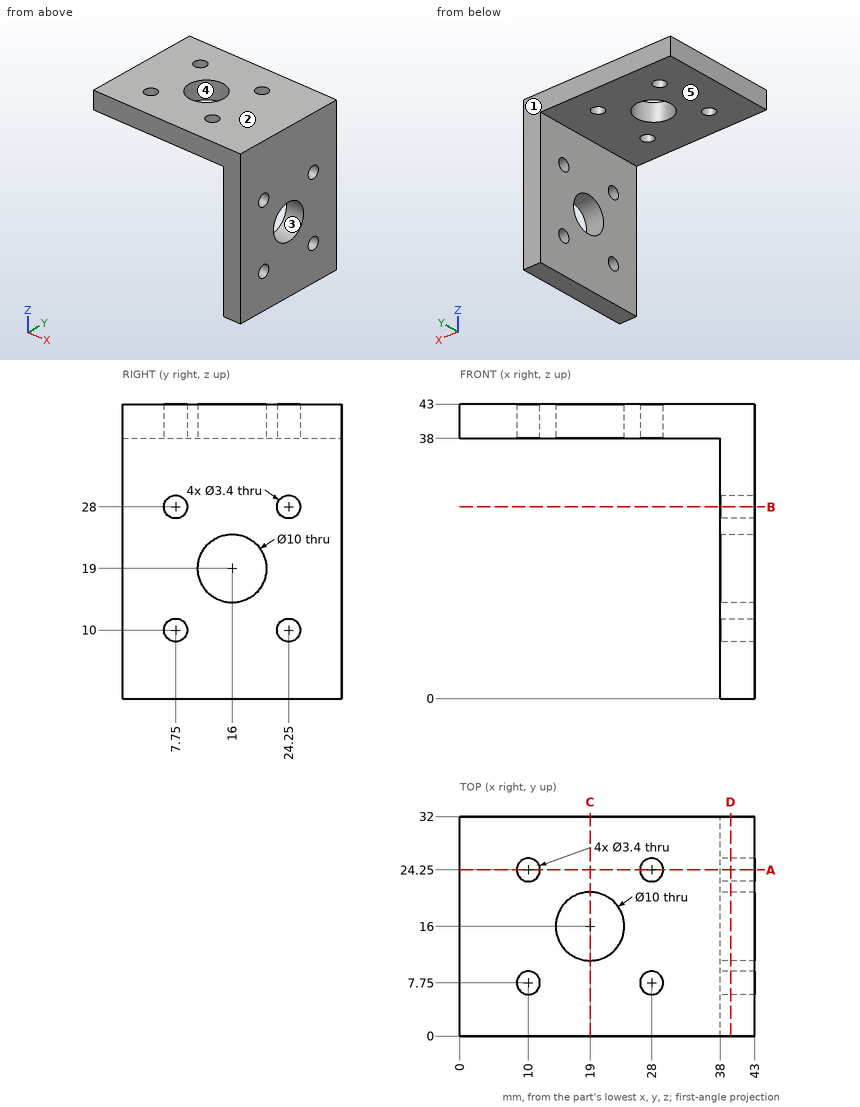
Design review of the part shown in the three views and the two pictorial views. Dimensions are in mm from the part's minimum x, y and z. A direction names the side the tool comes from. Coordinates: 2 decimals unless noted, no trailing zeros. Write each loop counter-clockwise with the first axis right and the second up, starting at its lowest first coordinate (ties: lowest second). Pieces come first, ordered by that corner, then holes. Notation, with made-up numbers: (28, 69.25) -> (51, 69.25) arc R26 ccw to (51, 101.25) -> close; hole circle Ø10 at (43, -23.5). An arc over 180 degrees is marked (long way). Answer in a Markdown table with one row per item.
1. We need section B-B, the plane z = 28. State the section outline as (x, y) points, and give its area (3 significant figures).
Answers below:
| item | result |
|---|---|
| outline | (38, 0) -> (43, 0) -> (43, 6.05) -> (38, 6.05) -> close; (38, 9.45) -> (43, 9.45) -> (43, 22.55) -> (38, 22.55) -> close; (38, 25.95) -> (43, 25.95) -> (43, 32) -> (38, 32) -> close |
| area | 126 mm^2 |
2. We need section C-C, the plane x = 19. State the section outline as (y, z) points, and give its area (3 significant figures).
Answers below:
| item | result |
|---|---|
| outline | (0, 38) -> (11, 38) -> (11, 43) -> (0, 43) -> close; (21, 38) -> (32, 38) -> (32, 43) -> (21, 43) -> close |
| area | 110 mm^2 |
3. For the marked faces 4 and 5, list the 3-axis set-ups (+Z, -Z, +X, -X, +Y, -Y) from which the entire face can be reached by the end or side of a thin tool; tool diameter is ignored.
Answers below:
| item | result |
|---|---|
| face 4 | +Z, -Z |
| face 5 | -Z, -X, +Y, -Y |
4. We need section D-D, the plane x = 39.5. State the section outline as (y, z) points, and give its area (3 significant figures).
Answers below:
| item | result |
|---|---|
| outline | (0, 0) -> (32, 0) -> (32, 43) -> (0, 43) -> close; hole circle Ø3.4 at (7.75, 10); hole circle Ø3.4 at (7.75, 28); hole circle Ø10 at (16, 19); hole circle Ø3.4 at (24.25, 10); hole circle Ø3.4 at (24.25, 28) |
| area | 1,260 mm^2 |
5. Wall thickness on probe 1 along Y at (x, z) = (28, 39.5); probe 2 along Y at (x, z) = (19, 40); probe 3 along Z at (x, y) = (24.5, 23.5): over which ranges is each line inside the solid? List them lowest first. Write a range as [from, to].
Answers below:
| item | result |
|---|---|
| probe 1 | y = [0, 6.05], [9.45, 22.55], [25.95, 32] |
| probe 2 | y = [0, 11], [21, 32] |
| probe 3 | z = [38, 43] |
6. We need section A-A, the plane y = 24.25. State the section outline as (x, z) points.
Answers below:
| item | result |
|---|---|
| outline | (0, 38) -> (8.3, 38) -> (8.3, 43) -> (0, 43) -> close; (11.7, 38) -> (26.3, 38) -> (26.3, 43) -> (11.7, 43) -> close; (29.7, 38) -> (38, 38) -> (38, 29.7) -> (43, 29.7) -> (43, 43) -> (29.7, 43) -> close; (38, 0) -> (43, 0) -> (43, 8.3) -> (38, 8.3) -> close; (38, 11.7) -> (43, 11.7) -> (43, 26.3) -> (38, 26.3) -> close |
7. Clearance check with flat-ended pins moving along their axes: pin 1 Ø6 at (x, y) = (27.5, 28) entering from -Z; pin 2 Ø2 at (y, z) = (15, 8) entering from -X. State where each tip first meets the part, or that it passes through.
Answers below:
| item | result |
|---|---|
| pin 1 | stops at z = 38 |
| pin 2 | stops at x = 38 |
8. Draft analysis for pull direction Z (two halves, no side actions). For the marked faces 1, 2 and 3, state which applies: +Z half, -Z half, draft (parallel to the pull), parting line (faces both ways), or undercut.
Answers below:
| item | result |
|---|---|
| face 1 | draft |
| face 2 | +Z half |
| face 3 | undercut |
